from build123d import *

# Parameters (mm, degrees)
CYLINDER003_R               = 3.5
CYLINDER003_DEPTH           = 10
CYLINDER002_R               = 2
CYLINDER002_DEPTH           = 10
FUSION_PITCH_ANGLE          = -90
CYLINDER_R                  = 15.5
CYLINDER_DEPTH              = 9
CYLINDER001_W               = 17.5
CYLINDER001_H               = 9
CYLINDER001_ANGLE           = 355
CYLINDER001_PLACEMENT_ANGLE = 182.5
BOX001_W                    = 5
BOX001_H                    = 30
BOX001_DEPTH                = 20
BOX_W                       = 24
BOX_H                       = 30
BOX_DEPTH                   = 9
CHAMFER_SIZE                = 10.9


with BuildPart() as cylinder003:
    # Cylinder003 → Cylinder003 (new body)
    with BuildSketch(Plane(origin=(15, -5, 5), x_dir=(1, 0, 0), z_dir=(0, 0, 1))):
        Circle(CYLINDER003_R)
    extrude(amount=CYLINDER003_DEPTH)


with BuildPart() as cone:
    # Cone → Cone (revolve)
    with BuildSketch(Plane(origin=(15, -5, 3), x_dir=(1, 0, 0), z_dir=(0, -1, 0))):
        Polygon((0, 0), (2, 0), (3.5, 2), (0, 2), align=None)
    revolve(axis=Axis((15, -5, 3), (0, 0, 1)))


with BuildPart() as fusion:
    # Cylinder002 → Cylinder002 (new body)
    with BuildSketch(Plane(origin=(15, -5, 0), x_dir=(1, 0, 0), z_dir=(0, 0, 1))):
        Circle(CYLINDER002_R)
    extrude(amount=CYLINDER002_DEPTH)

    # Fusion: union Cylinder003, Cone
    add(cylinder003.part)
    add(cone.part)


with BuildPart() as fusion_1:
    # Fusion pitch: moved
    add(fusion.part.rotate(Axis((0, 0, 0), (0, 1, 0)), FUSION_PITCH_ANGLE))


with BuildPart() as fusion_2:
    # Fusion placement: moved
    add(fusion_1.part.moved(Location((38, 5, 0))))


with BuildPart() as fusion002:
    # Cylinder → Cylinder (new body)
    with BuildSketch(Plane.XY):
        Circle(CYLINDER_R)
    extrude(amount=CYLINDER_DEPTH)

    # Fusion002: union Fusion
    add(fusion_2.part)


with BuildPart() as cylinder001:
    # Cylinder001 → Cylinder001 (revolve)
    with BuildSketch(Plane.XZ):
        with Locations((8.75, 4.5)):
            Rectangle(CYLINDER001_W, CYLINDER001_H)
    revolve(axis=Axis((0, 0, 0), (0, 0, 1)), revolution_arc=CYLINDER001_ANGLE)


with BuildPart() as cylinder001_1:
    # Cylinder001 placement: moved
    add(cylinder001.part.rotate(Axis((0, 0, 0), (0, 0, 1)), CYLINDER001_PLACEMENT_ANGLE))


with BuildPart() as cube001:
    # Box001 → Box001 (new body)
    with BuildSketch(Plane(origin=(32, -15, 0), x_dir=(1, 0, 0), z_dir=(0, 0, 1))):
        with Locations((2.5, 15)):
            Rectangle(BOX001_W, BOX001_H)
    extrude(amount=BOX001_DEPTH)


with BuildPart() as cut:
    # Box → Box (new body)
    with BuildSketch(Plane(origin=(8, -15, 0), x_dir=(1, 0, 0), z_dir=(0, 0, 1))):
        with Locations((12, 15)):
            Rectangle(BOX_W, BOX_H)
    extrude(amount=BOX_DEPTH)

    # Fusion003: union Cube001
    add(cube001.part)

    # Chamfer
    chamfer_edges = [cut.edges().sort_by_distance(p)[0] for p in [
        (32, 0, 9),
    ]]
    chamfer(chamfer_edges, length=CHAMFER_SIZE)

    # Fusion004: union Cylinder001
    add(cylinder001_1.part)

    # Cut: cut Fusion002
    add(fusion002.part, mode=Mode.SUBTRACT)


solid = cut.part
Verification items for the finished model (mm, model axes). A direction names the side the tool comes from. Coordinates: 2 decimals unless noted, no trailing zeros. Write each loop counter-clockwise with the first axis right and the second up, starting at its lowest first coordinate (ties: lowest second). Pieces come first, ordered by that corner, then holes. Notation, with made-up numbers: M 37.25,7.5 L 62.25,7.5 A28 cw 62.25,45.5 Z; hole C 3.25,12 d11. An arc over 180 degrees is marked long. Use a Markdown table: item, result.
Q1. Sectioned sample at D-D, the plane x = -11. Record the boundary of the cut face in (y, z), plus the area to 3 significant figures.
Reply:
| item | result |
|---|---|
| outline | M -13.61,0 L -10.92,0 L -10.92,9 L -13.61,9 Z; M 10.92,0 L 13.61,0 L 13.61,9 L 10.92,9 Z |
| area | 48.4 mm² |
Q2. Sectioned sample at C-C, the plane y = -9. Record the boundary of the cut face in (x, z), plus the area to 3 significant figures.
Reply:
| item | result |
|---|---|
| outline | M -15.01,0 L -12.62,0 L -12.62,9 L -15.01,9 Z; M 12.62,0 L 37,0 L 37,20 L 32,20 L 32,19.9 L 21.1,9 L 12.62,9 Z |
| area | 355 mm² |
Q3. Set-up check for faces 4 (the face through (26, -15, 8)), 5 (the face through (29.355, 0.154, 11.503)), 6 (the face through (-16.47, -0.72, 4.56)), 7 (the face through (15.3, -3.3, 9)): record each of +Z, -Z, +X, -X, +Y, -Y from which the full face is reachable in a straight line by a thin tool's end or side.
Reply:
| item | result |
|---|---|
| face 4 | +Z, -Z, +X, -Y |
| face 5 | -X |
| face 6 | +Z, -Z, -X |
| face 7 | +Z, -X, +Y, -Y |
Q4. Sectioned sample at A-A, the plane z = 15. Record the boundary of the cut face in (x, y), plus the area to 3 significant figures.
Reply:
| item | result |
|---|---|
| outline | M 27.1,-15 L 37,-15 L 37,-2 L 35,-2 L 33,-3.5 L 27.1,-3.5 Z; M 27.1,3.5 L 33,3.5 L 35,2 L 37,2 L 37,15 L 27.1,15 Z |
| area | 237 mm² |
Q5. Sectioned sample at B-B, the plane x = 0. Record the boundary of the cut face in (y, z), plus the area to 3 significant figures.
Reply:
| item | result |
|---|---|
| outline | M -17.5,0 L -15.5,0 L -15.5,9 L -17.5,9 Z; M 15.5,0 L 17.5,0 L 17.5,9 L 15.5,9 Z |
| area | 36.0 mm² |
Q6. Draft check along Y on faces 1 (the face through (-16.47, 0.72, 4.56)), 2 (the face through (25.3, -3.5, 13.2)), 3 (the face through (26, 15, 8)). Enter one of: +Y half, -Y half, draft (parallel to the pull), parting line (faces both ways), or undercut.
Reply:
| item | result |
|---|---|
| face 1 | undercut |
| face 2 | draft |
| face 3 | +Y half |
Q7. Thickness scan on line 1 (Z direction, x = 35.4, y = 0); line 2 (Y direction, x = 36.1, z = 15); line 3 (Y direction, x = 30.25, z = 15). Record the ranges inside material, lowest first.
Reply:
| item | result |
|---|---|
| line 1 | z = 0 to 13, 17 to 20 |
| line 2 | y = -15 to -2, 2 to 15 |
| line 3 | y = -15 to -3.5, 3.5 to 15 |
Q8. Go/stop test with flat-tipped pins: P1, Ø4.5, axis at y = 0, z = 15, coming from the -X side; P2, Ø4, axis at x = 27, z = 6.5, coming from the +Y side; P3, Ø6.5, axis at y = 0, z = 15, coming from the -X side; P4, Ø10, axis at x = -1.5, y = 11, coming from the -Z side. Record where each tip stops, or that it passes through.
Reply:
| item | result |
|---|---|
| P1 | stops at x = 34.67 |
| P2 | stops at y = 15 |
| P3 | stops at x = 33.33 |
| P4 | stops at z = 0 |
